Can you work these out from the model? Positions are in its coordinate system, mm. A direction names the side the tool comes from. Coordinates: 2 decimals unless noted, no trailing zeros. Write each loop counter-clockwise with the first axis right and the second up, starting at its lowest first coordinate (ties: lowest second). Pieces come first, ordered by that corner, then holes. Notation, with made-up numbers: M 37,31.5 L 57,31.5 A20 ccw 57,50.5 Z; hole C -6.5,4.5 d9. An arc over 180 degrees is marked long. Use one line per item in the form item = value. Start each with the question number.
```python
from build123d import *

# Parameters (mm, degrees)
BOX771_W                     = 6
BOX771_H                     = 6
BOX771_DEPTH                 = 2
BOX772_W                     = 6
BOX772_H                     = 6
BOX772_DEPTH                 = 2
BOX772_PLACEMENT_ANGLE       = 135
BOX769_W                     = 6
BOX769_H                     = 6
BOX769_DEPTH                 = 2
BOX767_W                     = 6
BOX767_H                     = 6
BOX767_DEPTH                 = 2
BOX767_PLACEMENT_ANGLE       = 225
BOX770_W                     = 6
BOX770_H                     = 6
BOX770_DEPTH                 = 2
BOX768_W                     = 6
BOX768_H                     = 6
BOX768_DEPTH                 = 2
BOX768_PLACEMENT_ANGLE       = 45
BOX773_W                     = 6
BOX773_H                     = 6
BOX773_DEPTH                 = 2
BOX765_W                     = 6
BOX765_H                     = 6
BOX765_DEPTH                 = 2
BOX765_PLACEMENT_ANGLE       = 45
CYLINDER1989_R               = 1.5
CYLINDER1989_DEPTH           = 10
CYLINDER1977_R               = 1.5
CYLINDER1977_DEPTH           = 10
CYLINDER1977_PLACEMENT_ANGLE = 135
CYLINDER1975_R               = 1.5
CYLINDER1975_DEPTH           = 10
CYLINDER1974_R               = 1.5
CYLINDER1974_DEPTH           = 10
CYLINDER1974_PLACEMENT_ANGLE = 225
CYLINDER1982_R               = 1.5
CYLINDER1982_DEPTH           = 10
CYLINDER1972_R               = 1.5
CYLINDER1972_DEPTH           = 10
CYLINDER1972_PLACEMENT_ANGLE = 45
CYLINDER1979_R               = 1.5
CYLINDER1979_DEPTH           = 10
CYLINDER1984_R               = 1.5
CYLINDER1984_DEPTH           = 10
CYLINDER1984_PLACEMENT_ANGLE = 45
CYLINDER1980_R               = 2.2
CYLINDER1980_DEPTH           = 10
TORUS004_R                   = 2.2
TUBE104_R                    = 35
TUBE104_R_2                  = 29
TUBE104_DEPTH                = 20


with BuildPart() as krychle771:
    # Box771 → Box771 (new body)
    with BuildSketch(Plane(origin=(-29, -3, 14), x_dir=(0, 1, 0), z_dir=(0, 0, 1))):
        with Locations((3, 3)):
            Rectangle(BOX771_W, BOX771_H)
    extrude(amount=BOX771_DEPTH)


with BuildPart() as krychle772:
    # Box772 → Box772 (new body)
    with BuildSketch(Plane.XY):
        with Locations((3, 3)):
            Rectangle(BOX772_W, BOX772_H)
    extrude(amount=BOX772_DEPTH)


with BuildPart() as krychle772_1:
    # Box772 placement: moved
    add(krychle772.part.moved(Location((-18.384776, -22.627417, 14))).rotate(Axis((-18.384776, -22.627417, 14), (0, 0, 1)), BOX772_PLACEMENT_ANGLE))


with BuildPart() as krychle769:
    # Box769 → Box769 (new body)
    with BuildSketch(Plane(origin=(3, -29, 14), x_dir=(-1, 0, 0), z_dir=(0, 0, 1))):
        with Locations((3, 3)):
            Rectangle(BOX769_W, BOX769_H)
    extrude(amount=BOX769_DEPTH)


with BuildPart() as krychle767:
    # Box767 → Box767 (new body)
    with BuildSketch(Plane.XY):
        with Locations((3, 3)):
            Rectangle(BOX767_W, BOX767_H)
    extrude(amount=BOX767_DEPTH)


with BuildPart() as krychle767_1:
    # Box767 placement: moved
    add(krychle767.part.moved(Location((22.627417, -18.384776, 14))).rotate(Axis((22.627417, -18.384776, 14), (0, 0, 1)), BOX767_PLACEMENT_ANGLE))


with BuildPart() as krychle770:
    # Box770 → Box770 (new body)
    with BuildSketch(Plane(origin=(29, 3, 14), x_dir=(0, -1, 0), z_dir=(0, 0, 1))):
        with Locations((3, 3)):
            Rectangle(BOX770_W, BOX770_H)
    extrude(amount=BOX770_DEPTH)


with BuildPart() as krychle768:
    # Box768 → Box768 (new body)
    with BuildSketch(Plane.XY):
        with Locations((3, 3)):
            Rectangle(BOX768_W, BOX768_H)
    extrude(amount=BOX768_DEPTH)


with BuildPart() as krychle768_1:
    # Box768 placement: moved
    add(krychle768.part.moved(Location((18.384776, 22.627417, 14))).rotate(Axis((18.384776, 22.627417, 14), (0, 0, -1)), BOX768_PLACEMENT_ANGLE))


with BuildPart() as krychle773:
    # Box773 → Box773 (new body)
    with BuildSketch(Plane(origin=(-3, 29, 14), x_dir=(1, 0, 0), z_dir=(0, 0, 1))):
        with Locations((3, 3)):
            Rectangle(BOX773_W, BOX773_H)
    extrude(amount=BOX773_DEPTH)


with BuildPart() as compound936:
    # Box765 → Box765 (new body)
    with BuildSketch(Plane.XY):
        with Locations((3, 3)):
            Rectangle(BOX765_W, BOX765_H)
    extrude(amount=BOX765_DEPTH)


with BuildPart() as compound936_1:
    # Box765 placement: moved
    add(compound936.part.moved(Location((-22.627417, 18.384776, 14))).rotate(Axis((-22.627417, 18.384776, 14), (0, 0, 1)), BOX765_PLACEMENT_ANGLE))

    # Compound936: union Krychle771, Krychle772, Krychle769, Krychle767, Krychle770, Krychle768, Krychle773
    add(krychle771.part)
    add(krychle772_1.part)
    add(krychle769.part)
    add(krychle767_1.part)
    add(krychle770.part)
    add(krychle768_1.part)
    add(krychle773.part)


with BuildPart() as obj1:
    # Cylinder1989 → Cylinder1989 (new body)
    with BuildSketch(Plane(origin=(-32, 0, 10), x_dir=(0, 1, 0), z_dir=(0, 0, 1))):
        Circle(CYLINDER1989_R)
    extrude(amount=CYLINDER1989_DEPTH)


with BuildPart() as obj2:
    # Cylinder1977 → Cylinder1977 (new body)
    with BuildSketch(Plane.XY):
        Circle(CYLINDER1977_R)
    extrude(amount=CYLINDER1977_DEPTH)


with BuildPart() as obj2_1:
    # Cylinder1977 placement: moved
    add(obj2.part.moved(Location((-22.627417, -22.627417, 10))).rotate(Axis((-22.627417, -22.627417, 10), (0, 0, 1)), CYLINDER1977_PLACEMENT_ANGLE))


with BuildPart() as obj3:
    # Cylinder1975 → Cylinder1975 (new body)
    with BuildSketch(Plane(origin=(0, -32, 10), x_dir=(-1, 0, 0), z_dir=(0, 0, 1))):
        Circle(CYLINDER1975_R)
    extrude(amount=CYLINDER1975_DEPTH)


with BuildPart() as obj4:
    # Cylinder1974 → Cylinder1974 (new body)
    with BuildSketch(Plane.XY):
        Circle(CYLINDER1974_R)
    extrude(amount=CYLINDER1974_DEPTH)


with BuildPart() as obj4_1:
    # Cylinder1974 placement: moved
    add(obj4.part.moved(Location((22.627417, -22.627417, 10))).rotate(Axis((22.627417, -22.627417, 10), (0, 0, 1)), CYLINDER1974_PLACEMENT_ANGLE))


with BuildPart() as obj5:
    # Cylinder1982 → Cylinder1982 (new body)
    with BuildSketch(Plane(origin=(32, 0, 10), x_dir=(0, -1, 0), z_dir=(0, 0, 1))):
        Circle(CYLINDER1982_R)
    extrude(amount=CYLINDER1982_DEPTH)


with BuildPart() as obj6:
    # Cylinder1972 → Cylinder1972 (new body)
    with BuildSketch(Plane.XY):
        Circle(CYLINDER1972_R)
    extrude(amount=CYLINDER1972_DEPTH)


with BuildPart() as obj6_1:
    # Cylinder1972 placement: moved
    add(obj6.part.moved(Location((22.627417, 22.627417, 10))).rotate(Axis((22.627417, 22.627417, 10), (0, 0, -1)), CYLINDER1972_PLACEMENT_ANGLE))


with BuildPart() as obj7:
    # Cylinder1979 → Cylinder1979 (new body)
    with BuildSketch(Plane(origin=(0, 32, 10), x_dir=(1, 0, 0), z_dir=(0, 0, 1))):
        Circle(CYLINDER1979_R)
    extrude(amount=CYLINDER1979_DEPTH)


with BuildPart() as compound938:
    # Cylinder1984 → Cylinder1984 (new body)
    with BuildSketch(Plane.XY):
        Circle(CYLINDER1984_R)
    extrude(amount=CYLINDER1984_DEPTH)


with BuildPart() as compound938_1:
    # Cylinder1984 placement: moved
    add(compound938.part.moved(Location((-22.627417, 22.627417, 10))).rotate(Axis((-22.627417, 22.627417, 10), (0, 0, 1)), CYLINDER1984_PLACEMENT_ANGLE))

    # Compound938: union obj1, obj2, obj3, obj4, obj5, obj6, obj7
    add(obj1.part)
    add(obj2_1.part)
    add(obj3.part)
    add(obj4_1.part)
    add(obj5.part)
    add(obj6_1.part)
    add(obj7.part)


with BuildPart() as compound938_2:
    # Compound938 placement: moved
    add(compound938_1.part.moved(Location((0, 0, -2))))


with BuildPart() as obj8:
    # Cylinder1980 → Cylinder1980 (new body)
    with BuildSketch(Plane(origin=(28, 0, 20.5), x_dir=(1, 0, 0), z_dir=(0, 0, 1))):
        Circle(CYLINDER1980_R)
    extrude(amount=CYLINDER1980_DEPTH)


with BuildPart() as obj9:
    # Torus004 → Torus004 (revolve)
    with BuildSketch(Plane(origin=(0, 0, 20.5), x_dir=(1, 0, 0), z_dir=(0, -1, 0))):
        with Locations((28.15, 0)):
            Circle(TORUS004_R)
    revolve(axis=Axis((0, 0, 20.5), (0, 0, 1)))


with BuildPart() as obj10:
    # Tube104 → Tube104 (new body)
    with BuildSketch(Plane.XY.offset(10)):
        Circle(TUBE104_R)
        Circle(TUBE104_R_2, mode=Mode.SUBTRACT)
    extrude(amount=TUBE104_DEPTH)

    # Cut598: cut obj9
    add(obj9.part, mode=Mode.SUBTRACT)

    # Cut599: cut obj8
    add(obj8.part, mode=Mode.SUBTRACT)

    # Cut597: cut Compound938
    add(compound938_2.part, mode=Mode.SUBTRACT)

    # Cut593: cut Compound936
    add(compound936_1.part, mode=Mode.SUBTRACT)


solid = obj10.part
```
1) Please list where these lines run through material, in increasing order: line 1 (X direction, y = 0, z = 17.3); line 2 (Y direction, x = -23, z = 11.25); line 3 (Y direction, x = -15, z = 24.5).
2) Suppose I cut it at A-A on z = 13. State how many separate pieces and enclosed holes the cut face has, and give its area (3 significant figures).
3) Will these pins go through, and if not, where does the flat tip stop? pin 1 Ø1.6 at (x, z) = (-32.5, 15) entering from +Y; pin 2 Ø1 at (x, z) = (-25.5, 16.5) entering from -Y; pin 3 Ø0.9 at (x, y) = (22, 22.5) entering from -Z.
4) Suppose I cut it at B-B on x = -32. Please give me the cut outline in (y, z).
5) Suppose I cut it at C-C on z = 25.5. Please give me the cut outline in (x, y).
6) If we mould it in two halves opening along Z, with no side actions, what happens to faces 5 (the face through (-5, 29, 10)), 6 (the face through (-30.536, -0.325, 11.972)), 7 (the face through (33.4, 1.4, 14))? For each: +Z half, -Z half, draft (parallel to the pull), parting line (faces both ways), or undercut.
7) Which directions (+Z, -Z, +X, -X, +Y, -Y) give clear straight access to the entire face, cutting with the end or side of a thin tool? Please do faces 1 (the face through (-24.67, 20.43, 14.99)), 2 (the face through (-24.67, -20.43, 14.99)), 3 (the face through (20.43, 24.67, 14.99)), 4 (the face through (23, -23, 18)).
Computed values:
q1.line_1 = -35 to -33.5, -30.5 to -29, 29 to 30.5, 33.5 to 35
q1.line_2 = -26.38 to -24.08, -21.17 to -17.66, 17.66 to 21.17, 24.08 to 26.38
q1.line_3 = -31.62 to -24.82, 24.82 to 31.62
q2.separate_pieces = 1
q2.enclosed_holes = 9
q2.area = 1,150 mm²
q3.pin_1 = 14.84
q3.pin_2 = -24.49
q3.pin_3 = 18
q4.outline = M -14.18,10 L -1.5,10 L -1.5,14 L -3,14 L -3,16 L -1.5,16 L -1.5,18 L 1.5,18 L 1.5,16 L 3,16 L 3,14 L 1.5,14 L 1.5,10 L 14.18,10 L 14.18,30 L -14.18,30 Z
q5.outline = C 0,0 d70; hole M 28.93,-1.99 A2.2 ccw 28.93,1.99 A29 ccw long Z
q6.face_5 = -Z half
q6.face_6 = draft
q6.face_7 = undercut
q7.face_1 = +Y
q7.face_2 = -Y
q7.face_3 = +X
q7.face_4 = -Z
